Drawing for the job (mm, zero at the part's lowest x, y, z). Round coordinates to 2 decimals unless told otherwise and drop trailing zeros. Write each loop counter-clockwise with the first axis right and the second up, starting at its lowest first coordinate (ties: lowest second). Pieces come first, ordered by that corner, then holes.
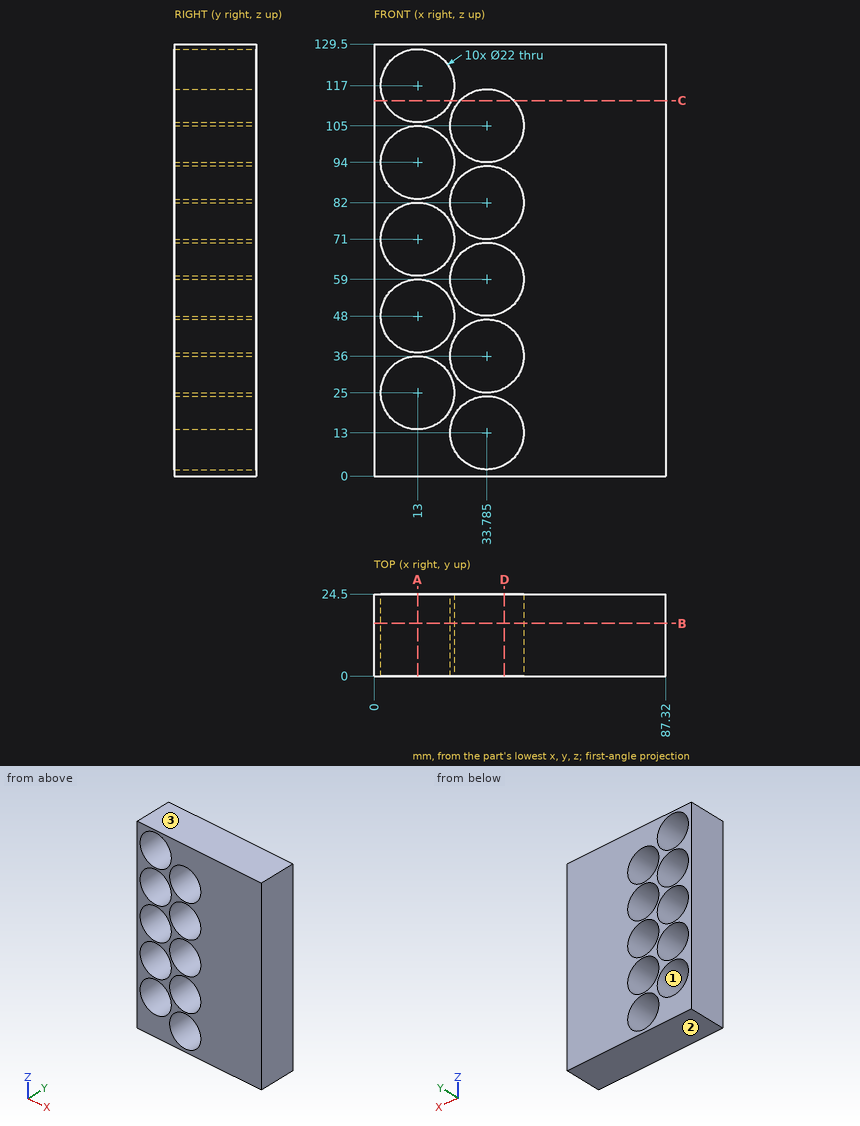
1) Cut at D-D on x = 39. List the corners of the cut face in (y, z) (1 decimal), and give its area (3 significant figures).
2) Cut at A-A on x = 13. List the corners of the cut face in (y, z).
3) Flat gauge pins, fed straight in: pin 1 Ø17.5 at (x, z) = (13, 94) entering from +Y; pin 2 Ø12 at (x, z) = (39, 81.5) entering from +Y. Where does each tip first touch, or does it go through?
4) Cut at C-C on z = 112.5. List the corners of the cut face in (x, y).
5) Wall check: probe 1 along Z at (x, y) = (33, 20); probe 2 along Z at (x, y) = (13, 10); probe 3 along X at (y, z) = (7.5, 19) (1 decimal). Give the ranges that are in metal, low to high.
6) Cut at B-B on y = 15.75. Give the number of separate pieces and of enclosed holes in the cut face, and give its area (3 significant figures).
7) Pull direction Z, two halves, no side cores. Call the marked faces 1, 2 and 3: released by +Z, released by -Z, zero draft, split by the parting line, or undercut.
Result sheet:
1. outline: (0, 0) - (24.5, 0) - (24.5, 3.3) - (0, 3.3) - close; (0, 22.7) - (24.5, 22.7) - (24.5, 26.3) - (0, 26.3) - close; (0, 45.7) - (24.5, 45.7) - (24.5, 49.3) - (0, 49.3) - close; (0, 68.7) - (24.5, 68.7) - (24.5, 72.3) - (0, 72.3) - close; (0, 91.7) - (24.5, 91.7) - (24.5, 95.3) - (0, 95.3) - close; (0, 114.7) - (24.5, 114.7) - (24.5, 129.5) - (0, 129.5) - close
1. area: 800 mm2
2. outline: (0, 0) - (24.5, 0) - (24.5, 14) - (0, 14) - close; (0, 36) - (24.5, 36) - (24.5, 37) - (0, 37) - close; (0, 59) - (24.5, 59) - (24.5, 60) - (0, 60) - close; (0, 82) - (24.5, 82) - (24.5, 83) - (0, 83) - close; (0, 105) - (24.5, 105) - (24.5, 106) - (0, 106) - close; (0, 128) - (24.5, 128) - (24.5, 129.5) - (0, 129.5) - close
3. pin 1: passes through
3. pin 2: stops at y = 24.5
4. outline: (0, 0) - (2.96, 0) - (2.96, 24.5) - (0, 24.5) - close; (23.04, 0) - (25.74, 0) - (25.74, 24.5) - (23.04, 24.5) - close; (41.83, 0) - (87.32, 0) - (87.32, 24.5) - (41.83, 24.5) - close
5. probe 1: z = 0 to 2.03, 23.97 to 25.03, 46.97 to 48.03, 69.97 to 71.03, 92.97 to 94.03, 115.97 to 129.5
5. probe 2: z = 0 to 14, 36 to 37, 59 to 60, 82 to 83, 105 to 106, 128 to 129.5
5. probe 3: x = 0 to 3.8, 22.2 to 24.6, 43 to 87.3
6. separate pieces: 1
6. enclosed holes: 10
6. area: 7,510 mm2
7. face 1: undercut
7. face 2: released by -Z
7. face 3: released by +Z
